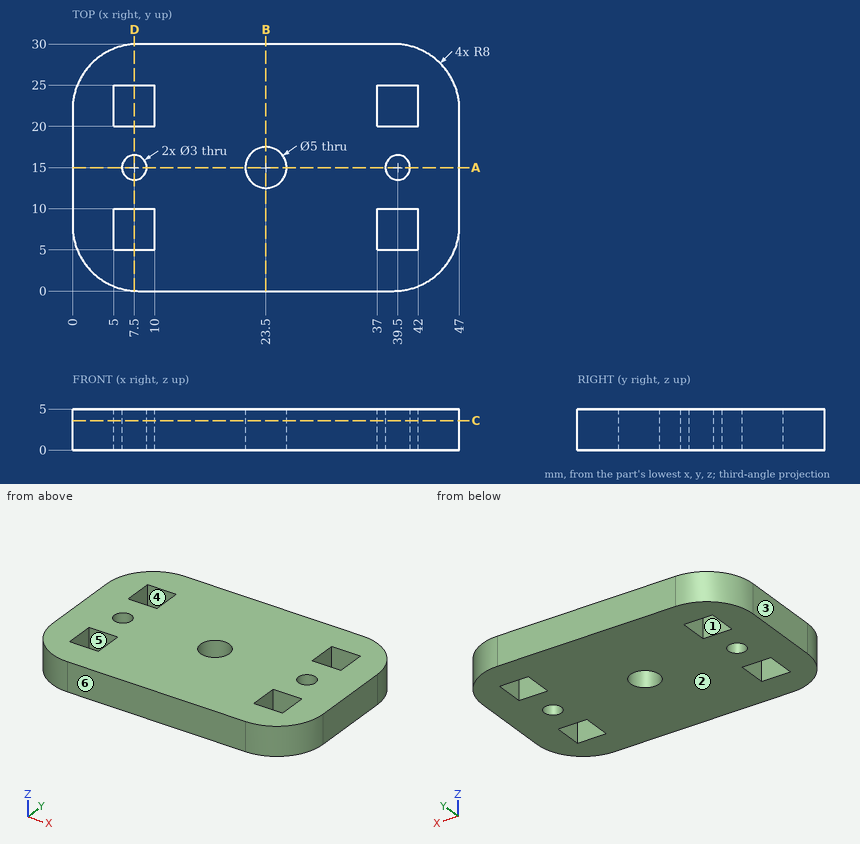
The drawing under review shows one solid part. Ordinate dimensions are in mm from its lowest x, y, z. A direction names the side the tool comes from. Round coordinates to 2 decimals unless told otherwise and drop trailing zeros. Loops run counter-clockwise (first coordinate to the right, second up) from the corner with the lowest first, then second, coordinate; pieces in that order, holes last.
Item 1: For the marked faces 5 and 6, list the 3-axis set-ups (+Z, -Z, +X, -X, +Y, -Y) from which the entire face can be reached by the end or side of a thin tool; tool diameter is ignored.
Determined:
face 5: +Z, -Z
face 6: +Z, -Z, +X, -X, -Y
Item 2: Take a section at B-B (x = 23.5). Write out the cut boundary in (y, z), then the cut area to 3 significant figures.
Determined:
outline: (0, 0) - (12.5, 0) - (12.5, 5) - (0, 5) - close; (17.5, 0) - (30, 0) - (30, 5) - (17.5, 5) - close
area: 125 mm2
Item 3: Mouldability with a two-part tool opening along X and no side actions: class the marked faces 1, 2, 3 and 4 as released by +X, released by -X, zero draft, split by the parting line, or undercut.
Determined:
face 1: undercut
face 2: zero draft
face 3: released by -X
face 4: undercut
Item 4: For line 1 (X direction, y = 21, z = 0.5); line 2 (Y direction, x = 37.5, z = 4.2); line 3 (Y direction, x = 39.5, z = 3.8), list the stretches that pass through material, from the lowest coordinate up.
Determined:
line 1: x = 0 to 5, 10 to 37, 42 to 47
line 2: y = 0 to 5, 10 to 20, 25 to 30
line 3: y = 0.02 to 5, 10 to 13.5, 16.5 to 20, 25 to 29.98
Item 5: Clearance check with a flat-ended pin moving along its axis: pin 1 Ø2.5 at (x, y) = (39.5, 15) entering from +Z. State where the tip first meets the part, or that it passes through.
Determined:
pin 1: passes through
Item 6: Take a section at C-C (z = 3.6). Write out the cut boundary in (x, y), then the cut area to 3 significant figures.
Determined:
outline: (0, 8) arc R8 ccw to (8, 0) - (39, 0) arc R8 ccw to (47, 8) - (47, 22) arc R8 ccw to (39, 30) - (8, 30) arc R8 ccw to (0, 22) - close; hole (5, 5) - (10, 5) - (10, 10) - (5, 10) - close; hole (5, 20) - (10, 20) - (10, 25) - (5, 25) - close; hole circle Ø3 at (7.5, 15); hole circle Ø5 at (23.5, 15); hole (37, 5) - (42, 5) - (42, 10) - (37, 10) - close; hole (37, 20) - (42, 20) - (42, 25) - (37, 25) - close; hole circle Ø3 at (39.5, 15)
area: 1,220 mm2
Item 7: Take a section at D-D (x = 7.5). Write out the cut boundary in (y, z), then the cut area to 3 significant figures.
Determined:
outline: (0.02, 0) - (5, 0) - (5, 5) - (0.02, 5) - close; (10, 0) - (13.5, 0) - (13.5, 5) - (10, 5) - close; (16.5, 0) - (20, 0) - (20, 5) - (16.5, 5) - close; (25, 0) - (29.98, 0) - (29.98, 5) - (25, 5) - close
area: 84.8 mm2
Item 8: Take a section at A-A (y = 15). Write out the cut boundary in (x, z).
Determined:
outline: (0, 0) - (6, 0) - (6, 5) - (0, 5) - close; (9, 0) - (21, 0) - (21, 5) - (9, 5) - close; (26, 0) - (38, 0) - (38, 5) - (26, 5) - close; (41, 0) - (47, 0) - (47, 5) - (41, 5) - close
